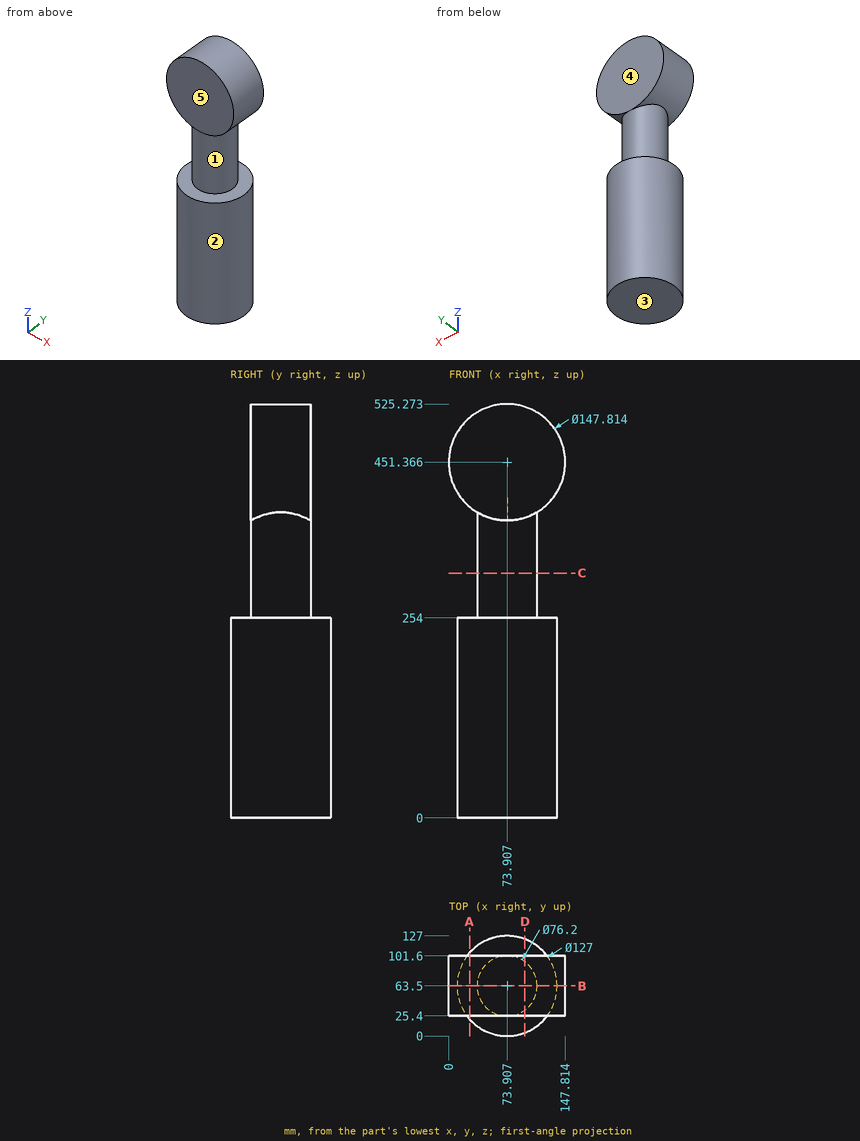
The figure shows three views and two pictorial views of one solid part (mm, origin at its lowest corner). Answer the questions. A direction names the side the tool comes from. Coordinates: 2 decimals unless noted, no trailing zeros. Write each loop counter-clockwise with the first axis right and the second up, starting at its lowest first coordinate (ties: lowest second). Pieces come first, ordered by that corner, then holes. Notation, with made-up numbers: M 45.5,3.5 L 98.5,3.5 A33 cw 98.5,32.5 Z; hole C 31,-33.75 d11. An arc over 180 degrees is marked long. Answer as CSV lines item,"result". Start each with the question number.
Item 1: Determine the mould class of the marked faces 1, 2 and 3 for opening direction Z: released by +Z, released by -Z, zero draft, split by the parting line, or undercut.
Item 2: Section A-A on x = 26.5 is taken. Write down the section's boundary in (y, z), and give its area (3 significant figures).
Item 3: Consider L1, parallel to Y at x = 126.5, z = 415.5; L2, parallel to X at y = 33, z = 489 (1 decimal); L3, parallel to Z at x = 54, y = 98. Determine where each line is inside the solid, lowest interval first.
Item 4: Flat-ended cylindrical pins translate along their axes: P1, Ø3, axis at y = 62, z = 77.5, coming from the +X side; P2, Ø2, axis at x = 20, z = 230, coming from the +Y side (1 decimal); P3, Ø4, axis at x = 125.5, y = 92.5, coming from the +Z side. Find the tip coordinate at first contact, or state that the pin passes through.
Item 5: Section B-B on y = 63.5 is taken. Write down the section's boundary in (x, z), and give its area (3 significant figures).
Item 6: Section D-D on x = 96.5 is taken. Write down the section's boundary in (y, z) (1 decimal), and give its area (3 significant figures).
Item 7: Section C-C on z = 310.5 is taken. Write down the section's boundary in (x, y), and give its area (3 significant figures).
Item 8: A tool of negligible diameter and unlimited length cuts with its end or side. For the marked faces 4 and 5, from which of +Z, -Z, +X, -X, +Y, -Y can it reach the whole face along a straight path? Write none if from no direction.
Checks:
1,face 1,"undercut"
1,face 2,"zero draft"
1,face 3,"released by -Z"
2,outline,"M 21.25,0 L 105.75,0 L 105.75,254 L 21.25,254 Z; M 25.4,394.67 L 101.6,394.67 L 101.6,508.07 L 25.4,508.07 Z"
2,area,"30,100 mm²"
3,L1,"y = 25.4 to 101.6"
3,L2,"x = 10.3 to 137.5"
3,L3,"z = 0 to 254, 380.19 to 522.54"
4,P1,"stops at x = 137.41"
4,P2,"stops at y = 98.6"
4,P3,"stops at z = 506.16"
5,outline,"M 10.41,0 L 137.41,0 L 137.41,254 L 112.01,254 L 112.01,388.04 A73.91 ccw long 35.81,388.04 L 35.81,254 L 10.41,254 Z"
5,area,"59,100 mm²"
6,outline,"M 4.2,0 L 122.8,0 L 122.8,254 L 94.2,254 L 94.2,381 L 101.6,381 L 101.6,521.7 L 25.4,521.7 L 25.4,381 L 32.8,381 L 32.8,254 L 4.2,254 Z"
6,area,"48,700 mm²"
7,outline,"C 73.91,63.5 d76.2"
7,area,"4,560 mm²"
8,face 4,"+Z, +X, -X, +Y"
8,face 5,"+Z, +X, -X, -Y"
